```python
from build123d import *

# Parameters (mm, degrees)
SKETCH1_W                    = 1343.025
SKETCH1_H                    = 527.05
BOSS_EXTRUDE1_DEPTH          = 17.78
FILLET1_R                    = 6.35
F_1_8_0_125_DIAMETER_HOLE1_D = 3.175
SKETCH5_W                    = 103.867264199
SKETCH5_H                    = 400.05
CUT_EXTRUDE1_DEPTH           = 722.588935393
CUT_EXTRUDE2_DEPTH           = 9.525
FILLET2_R                    = 6.35


with BuildPart() as part:
    # Sketch1 → Boss-Extrude1 (new body)
    with BuildSketch(Plane(origin=(0, 0, 0), x_dir=(1, 0, 0), z_dir=(0, 1, 0))):
        Rectangle(SKETCH1_W, SKETCH1_H)
    extrude(amount=BOSS_EXTRUDE1_DEPTH)

    # Fillet1
    fillet1_edges = [part.edges().sort_by_distance(p)[0] for p in [
        (671.5125, 8.89, 263.525),
        (-671.5125, 8.89, 263.525),
        (-671.5125, 8.89, -263.525),
        (671.5125, 8.89, -263.525),
    ]]
    fillet(fillet1_edges, radius=FILLET1_R)

    # 1/8 (0.125) Diameter Hole1 (through all)
    with Locations(Plane(origin=(0, 17.78, 0), x_dir=(1, 0, 0), z_dir=(0, 1, 0))):
        with Locations((0, 0), (457.2, 152.4), (-457.2, -152.4), (-457.2, 152.4), (457.2, -152.4)):
            Hole(F_1_8_0_125_DIAMETER_HOLE1_D / 2)

    # Sketch5 → Cut-Extrude1 (cut, through all)
    with BuildSketch(Plane(origin=(0, 17.78, 0), x_dir=(1, 0, 0), z_dir=(0, 1, 0))):
        Polygon((-406.4, 200.025), (406.4, 200.025), (0, 38.1), align=None)
        Polygon((0, -38.1), (-406.4, -200.025), (406.4, -200.025), align=None)
        Polygon((406.4, 146.74453125), (406.4, -146.74453125), (38.1, 0), align=None)
        Polygon((-406.4, 146.74453125), (-38.1, 0), (-406.4, -146.74453125), align=None)
        with Locations((556.0788679, 0)):
            Rectangle(SKETCH5_W, SKETCH5_H)
        with Locations((-556.0788679, 0)):
            Rectangle(SKETCH5_W, SKETCH5_H)
    extrude(amount=-CUT_EXTRUDE1_DEPTH, mode=Mode.SUBTRACT)

    # Sketch6 → Cut-Extrude2 (cut)
    with BuildSketch(Plane(origin=(0, 17.78, 0), x_dir=(1, 0, 0), z_dir=(0, 1, 0))):
        with BuildLine():
            Line((639.7625, -263.525), (665.1625, -263.525))
            ThreePointArc((665.1625, -263.525), (669.652628061, -261.665128061), (671.5125, -257.175))
            Line((671.5125, -257.175), (671.5125, 257.175))
            ThreePointArc((671.5125, 257.175), (669.652628061, 261.665128061), (665.1625, 263.525))
            Line((665.1625, 263.525), (639.7625, 263.525))
            Line((639.7625, 263.525), (639.7625, -263.525))
        make_face()
        with BuildLine():
            Line((-639.7625, -263.525), (-665.1625, -263.525))
            ThreePointArc((-665.1625, -263.525), (-669.652628061, -261.665128061), (-671.5125, -257.175))
            Line((-671.5125, -257.175), (-671.5125, 257.175))
            ThreePointArc((-671.5125, 257.175), (-669.652628061, 261.665128061), (-665.1625, 263.525))
            Line((-665.1625, 263.525), (-639.7625, 263.525))
            Line((-639.7625, 263.525), (-639.7625, -263.525))
        make_face()
    extrude(amount=-CUT_EXTRUDE2_DEPTH, mode=Mode.SUBTRACT)

    # Fillet2
    fillet2_edges = [part.edges().sort_by_distance(p)[0] for p in [
        (-504.145235801, 8.89, -200.025),
        (-504.145235801, 8.89, 200.025),
        (-608.0125, 8.89, 200.025),
        (-608.0125, 8.89, -200.025),
        (-406.4, 8.89, 146.74453125),
        (-406.4, 8.89, -146.74453125),
        (-38.1, 8.89, 0),
        (608.0125, 8.89, -200.025),
        (608.0125, 8.89, 200.025),
        (504.145235801, 8.89, 200.025),
        (504.145235801, 8.89, -200.025),
        (0, 8.89, 38.1),
        (406.4, 8.89, 200.025),
        (-406.4, 8.89, 200.025),
        (38.1, 8.89, 0),
        (406.4, 8.89, -146.74453125),
        (406.4, 8.89, 146.74453125),
        (639.7625, 13.0175, 263.525),
        (639.7625, 13.0175, -263.525),
        (-639.7625, 13.0175, -263.525),
        (-639.7625, 13.0175, 263.525),
        (406.4, 8.89, -200.025),
        (0, 8.89, -38.1),
        (-406.4, 8.89, -200.025),
    ]]
    fillet(fillet2_edges, radius=FILLET2_R)


solid = part.part
```
Source: CAD feature listing. Evaluate the final solid. Frame: model axes, mm. A direction names the side the tool comes from. Give positions to 0.01 mm unless a question says otherwise; leave off trailing zeros. Write each loop counter-clockwise with the first axis right and the second up, starting at its lowest first coordinate (ties: lowest second). Pieces come first, ordered by that corner, then holes. Notation, with made-up numbers: (-25.5, 2) - (-17.5, 2) arc R20 ccw to (-17.5, 33) - close; hole circle Ø8 at (33, 73.5). An arc over 180 degrees is marked (long way). One line per item, written item: value. Start each with the question number.
Q1. Set-up query: faces 1 (the face through (-9, 17.78, -4)), 2 (the face through (227.72, 9.01, 75.55)). Return all of +Z, -Z, +X, -X, +Y, -Y with unobstructed straight access to the full face (end or side cutting, diameter ignored); none if empty.
Q2. Draft query along X for faces 3 (the face through (-656, 8.255, -4)), 4 (the face through (-227.72, 9.01, -75.55)). Return one class per face: +X half, -X half, draft (parallel to the pull), parting line (faces both ways), or undercut.
Q3. Section query A-A, the plane x = 147. Return the cut outline in (y, z) (3 decimals), then the cut area to 3 significant figures.
Q4. First-contact query: pin 1 Ø5 at (y, z) = (15, -30) entering from -X. Flat tip, straight axial feed; report the tip coordinate or a pass-through.
Q5. Section query B-B, the plane y = 4. Count the separate pieces of the cut face and the enclosed holes in it, then the cut area to 3 significant figures.
Q6. Material intervals for probe 1 along Z at (x, y) = (0, 6.75) (1 decimal); probe 2 along Z at (x, y) = (-457.2, 5.25) (1 decimal); probe 3 along Z at (x, y) = (-263, 2) (3 decimals), sorted ascending. Write a range as from..to.
Answer:
1. face 1: +Z, -Z, +X, -X, +Y
1. face 2: +Y, -Y
2. face 3: draft
2. face 4: undercut
3. outline: (0, -263.525) - (17.78, -263.525) - (17.78, -200.025) - (0, -200.025) - close; (0, -96.67) - (17.78, -96.67) - (17.78, -43.39) - (0, -43.39) - close; (0, 43.39) - (17.78, 43.39) - (17.78, 96.67) - (0, 96.67) - close; (0, 200.025) - (17.78, 200.025) - (17.78, 263.525) - (0, 263.525) - close
3. area: 4,150 mm2
4. pin 1: stops at x = -639.76
5. separate pieces: 1
5. enclosed holes: 11
5. area: 386,000 mm2
6. probe 1: z = -263.5..-200, -38.6..-1.6, 1.6..38.6, 200..263.5
6. probe 2: z = -263.5..-154, -150.8..150.8, 154..263.5
6. probe 3: z = -263.525..-200.025, -142.889..-89.609, 89.609..142.889, 200.025..263.525
